Design review of the part built by this model. Coordinates are the model's own, in mm. A direction names the side the tool comes from. Coordinates: 2 decimals unless noted, no trailing zeros. Order: outer loops, then holes, each group sorted by start corner. A loop starts at its lowest first (then second) coordinate and runs counter-clockwise, first axis right, second up. Notation, with made-up numbers: M -13,70.5 L 41,70.5 A27 cw 41,102.5 Z; hole C 36,-16.5 d6. An arc over 180 degrees is marked long. Use CSV: the item, a comma, the result in double quotes.
```python
from build123d import *

# Parameters (mm, degrees)
F0_W     = 90
F0_H     = 126
F1_DEPTH = 25
F2_W     = 50
F2_H     = 65
F3_DEPTH = 30


with BuildPart() as f1:
    # F0 (on Front) → F1 (new body, symmetric)
    with BuildSketch(Plane.XZ):
        Rectangle(F0_W, F0_H)
    extrude(amount=F1_DEPTH, both=True)

    # F2 (on face) → F3 (join)
    with BuildSketch(Plane.XZ.offset(25)):
        with Locations((10, -20.5)):
            Rectangle(F2_W, F2_H)
    extrude(amount=F3_DEPTH)


solid = f1.part
```
(1) Add section C-C on y = -27. State the section outline as (x, z) points, and give its area (3 significant figures).
The answers:
outline,"M -15,-53 L 35,-53 L 35,12 L -15,12 Z"
area,"3,250 mm2"
(2) Add section B-B on x = 22.5. State the section outline as (y, z) points.
The answers:
outline,"M -55,-53 L -25,-53 L -25,-63 L 25,-63 L 25,63 L -25,63 L -25,12 L -55,12 Z"
(3) Add section A-A on z = -41.5. State the section outline as (x, y) points, and give its area (3 significant figures).
The answers:
outline,"M -45,-25 L -15,-25 L -15,-55 L 35,-55 L 35,-25 L 45,-25 L 45,25 L -45,25 Z"
area,"6,000 mm2"
(4) Add section D-D on x = -31.5. State the section outline as (y, z) points.
The answers:
outline,"M -25,-63 L 25,-63 L 25,63 L -25,63 Z"
(5) For faces 1 (the face through (10, -40, -53)), 2 (the face through (-15, -40, -21)), 3 (the face through (-1, 0, 63)), 4 (the face through (35, -40, -21)), 5 (the face through (10, -40, 12)), list the 3-axis set-ups (+Z, -Z, +X, -X, +Y, -Y) from which the entire face can be reached by the end or side of a thin tool; tool diameter is ignored.
The answers:
face 1,"-Z, +X, -X, -Y"
face 2,"+Z, -Z, -X, -Y"
face 3,"+Z, +X, -X, +Y, -Y"
face 4,"+Z, -Z, +X, -Y"
face 5,"+Z, +X, -X, -Y"
(6) Wall thickness on probe 1 along X at (y, z) = (-30.5, -30); probe 2 along Z at (x, y) = (-13.5, -43.5); probe 3 along Y at (x, z) = (38, -34.5): over which ranges is each line inside the solid? List them lowest first.
The answers:
probe 1,"x = -15 to 35"
probe 2,"z = -53 to 12"
probe 3,"y = -25 to 25"
(7) Clearance check with flat-ended pins moving along their axes: P1, Ø9, axis at y = -36, z = -34.5, coming from the +X side; P2, Ø15, axis at x = 9, y = -46.5, coming from the -Z side. State where each tip first meets the part, or that it passes through.
The answers:
P1,"stops at x = 35"
P2,"stops at z = -53"
